```python
from build123d import *

# Parameters (mm, degrees)
BOSS_EXTRUDE1_DEPTH     = 22.5
CUT_EXTRUDE1_DEPTH      = 17.5
SKETCH4_R               = 1
CUT_EXTRUDE2_DEPTH      = 15
CUT_EXTRUDE2_DEPTH_BACK = 12.5
SKETCH5_W               = 10.5
SKETCH5_H               = 12.5
CUT_EXTRUDE3_DEPTH      = 20
SKETCH6_R               = 1.4
CUT_EXTRUDE4_DEPTH      = 10
SKETCH8_R               = 1
SKETCH8_W               = 24
SKETCH8_H               = 13
CUT_EXTRUDE6_DEPTH      = 6
SKETCH9_R               = 1.5
CUT_EXTRUDE7_DEPTH      = 23.5
SKETCH10_R              = 3
CUT_EXTRUDE8_DEPTH      = 5
SKETCH14_W              = 12
SKETCH14_H              = 17.5
BOSS_EXTRUDE3_DEPTH     = 3.5
SKETCH11_R              = 1.5
CUT_EXTRUDE9_DEPTH      = 10
SKETCH16_R              = 2
CUT_EXTRUDE11_DEPTH     = 2
SKETCH18_W              = 6.5
SKETCH18_H              = 2.5
CUT_EXTRUDE12_DEPTH     = 23.5
CUT_EXTRUDE14_DEPTH     = 35
SKETCH22_R              = 1.6
CUT_EXTRUDE15_DEPTH     = 23.5
SKETCH23_R              = 3
CUT_EXTRUDE18_DEPTH     = 3
SKETCH25_W              = 5
SKETCH25_H              = 11.5
BOSS_EXTRUDE4_DEPTH     = 2


with BuildPart() as part:
    # Sketch2 → Boss-Extrude1 (new body)
    with BuildSketch(Plane(origin=(0, 0, 0), x_dir=(1, 0, 0), z_dir=(0, 1, 0))):
        with BuildLine():
            Line((0, 0), (46, 0))
            ThreePointArc((46, 0), (53.071067812, 2.928932188), (56, 10))
            Line((56, 10), (56, 24))
            ThreePointArc((56, 24), (53.071067812, 31.071067812), (46, 34))
            Line((46, 34), (0, 34))
            Line((0, 34), (0, 14))
            Line((0, 14), (-6.5, 14))
            Line((-6.5, 14), (-6.5, 0))
            Line((-6.5, 0), (0, 0))
        make_face()
    extrude(amount=BOSS_EXTRUDE1_DEPTH)

    # Sketch3 → Cut-Extrude1 (cut)
    with BuildSketch(Plane(origin=(0, 22.5, 0), x_dir=(1, 0, 0), z_dir=(0, 1, 0))):
        with BuildLine():
            Line((45, 32), (5, 32))
            Line((5, 32), (5, 3.5))
            Line((5, 3.5), (17, 3.5))
            Line((17, 3.5), (17, 2))
            Line((17, 2), (45, 2))
            Line((45, 2), (45, 4))
            ThreePointArc((45, 4), (46.464466094, 7.535533906), (50, 9))
            Line((50, 9), (54, 9))
            Line((54, 9), (54, 25))
            Line((54, 25), (50, 25))
            ThreePointArc((50, 25), (46.464466094, 26.464466094), (45, 30))
            Line((45, 30), (45, 32))
        make_face()
    extrude(amount=-CUT_EXTRUDE1_DEPTH, mode=Mode.SUBTRACT)

    # Sketch4 → Cut-Extrude2 (cut, two sides)
    with BuildSketch(Plane(origin=(5, 0, 0), x_dir=(0, 0, -1), z_dir=(1, 0, 0))) as cut_extrude2_sk:
        with Locations((28.5, 15.25)):
            Circle(SKETCH4_R)
        with Locations((28.5, 7.25)):
            Circle(SKETCH4_R)
        with Locations((16.5, 7.25)):
            Circle(SKETCH4_R)
        with Locations((16.5, 15.25)):
            Circle(SKETCH4_R)
    extrude(amount=CUT_EXTRUDE2_DEPTH, mode=Mode.SUBTRACT)
    extrude(cut_extrude2_sk.sketch, amount=-CUT_EXTRUDE2_DEPTH_BACK, mode=Mode.SUBTRACT)

    # Sketch5 → Cut-Extrude3 (cut)
    with BuildSketch(Plane.ZY.offset(6.5)):
        with Locations((-8.75, 11.5)):
            Rectangle(SKETCH5_W, SKETCH5_H)
    extrude(amount=-CUT_EXTRUDE3_DEPTH, mode=Mode.SUBTRACT)

    # Sketch6 → Cut-Extrude4 (cut)
    with BuildSketch(Plane(origin=(0, 22.5, 0), x_dir=(1, 0, 0), z_dir=(0, 1, 0))):
        with Locations((0.5, 10)):
            Circle(SKETCH6_R)
    extrude(amount=-CUT_EXTRUDE4_DEPTH, mode=Mode.SUBTRACT)

    # Sketch8 → Cut-Extrude6 (cut, through all)
    with BuildSketch(Plane(origin=(0, 5, 0), x_dir=(1, 0, 0), z_dir=(0, 1, 0))):
        with Locations((50.6, 17)):
            Circle(SKETCH8_R)
        with Locations((22.4, 17)):
            Circle(SKETCH8_R)
        with Locations((36.5, 17)):
            Rectangle(SKETCH8_W, SKETCH8_H)
    extrude(amount=-CUT_EXTRUDE6_DEPTH, mode=Mode.SUBTRACT)

    # Sketch9 → Cut-Extrude7 (cut, through all)
    with BuildSketch(Plane(origin=(0, 22.5, 0), x_dir=(1, 0, 0), z_dir=(0, 1, 0))):
        with Locations((49.5, 29)):
            Circle(SKETCH9_R)
        with Locations((49.5, 5)):
            Circle(SKETCH9_R)
    extrude(amount=-CUT_EXTRUDE7_DEPTH, mode=Mode.SUBTRACT)

    # Sketch10 → Cut-Extrude8 (cut)
    with BuildSketch(Plane.XZ):
        with Locations((49.5, -5)):
            Circle(SKETCH10_R)
        with Locations((49.5, -29)):
            Circle(SKETCH10_R)
    extrude(amount=-CUT_EXTRUDE8_DEPTH, mode=Mode.SUBTRACT)

    # Sketch14 → Boss-Extrude3 (add, symmetric)
    with BuildSketch(Plane.XY.offset(-22.5)):
        with Locations((11, 13.75)):
            Rectangle(SKETCH14_W, SKETCH14_H)
    extrude(amount=BOSS_EXTRUDE3_DEPTH, both=True)

    # Sketch11 → Cut-Extrude9 (cut)
    with BuildSketch(Plane.XZ):
        with Locations((8, -8)):
            Circle(SKETCH11_R)
        with Locations((8, -26)):
            Circle(SKETCH11_R)
    extrude(amount=-CUT_EXTRUDE9_DEPTH, mode=Mode.SUBTRACT)

    # Sketch16 → Cut-Extrude11 (cut)
    with BuildSketch(Plane(origin=(5, 0, 0), x_dir=(0, 0, -1), z_dir=(1, 0, 0))):
        with Locations((28.5, 15.25)):
            Circle(SKETCH16_R)
        with Locations((28.5, 7.25)):
            Circle(SKETCH16_R)
        with Locations((16.5, 7.25)):
            Circle(SKETCH16_R)
        with Locations((16.5, 15.25)):
            Circle(SKETCH16_R)
    extrude(amount=-CUT_EXTRUDE11_DEPTH, mode=Mode.SUBTRACT)

    # Sketch18 → Cut-Extrude12 (cut, through all)
    with BuildSketch(Plane(origin=(0, 22.5, 0), x_dir=(1, 0, 0), z_dir=(0, 1, 0))):
        with Locations((-3.25, 1.25)):
            Rectangle(SKETCH18_W, SKETCH18_H)
    extrude(amount=-CUT_EXTRUDE12_DEPTH, mode=Mode.SUBTRACT)

    # Sketch21 → Cut-Extrude14 (cut, through all)
    with BuildSketch(Plane.XY):
        Polygon((5, 22.5), (56, 11.25), (56, 22.5), align=None)
    extrude(amount=-CUT_EXTRUDE14_DEPTH, mode=Mode.SUBTRACT)

    # Sketch22 → Cut-Extrude15 (cut, through all)
    with BuildSketch(Plane.XZ):
        with Locations((14, -22.5)):
            Circle(SKETCH22_R)
    extrude(amount=-CUT_EXTRUDE15_DEPTH, mode=Mode.SUBTRACT)

    # Sketch23 → Cut-Extrude18 (cut)
    with BuildSketch(Plane.XZ):
        with Locations((14, -22.5)):
            Circle(SKETCH23_R)
    extrude(amount=-CUT_EXTRUDE18_DEPTH, mode=Mode.SUBTRACT)

    # Sketch25 → Boss-Extrude4 (add)
    with BuildSketch(Plane(origin=(0, 22.5, 0), x_dir=(1, 0, 0), z_dir=(0, 1, 0))):
        with Locations((-4, 8.25)):
            Rectangle(SKETCH25_W, SKETCH25_H)
    extrude(amount=BOSS_EXTRUDE4_DEPTH)


solid = part.part
```
Geometry: final body of the model. Coordinates: model frame, mm. A direction names the side the tool comes from. Round coordinates to 2 decimals unless told otherwise and drop trailing zeros. Loops run counter-clockwise (first coordinate to the right, second up) from the corner with the lowest first, then second, coordinate; pieces in that order, holes last. Notation, with made-up numbers: (20.25, 46.5) -> (35.25, 46.5) arc R33 ccw to (35.25, 84.5) -> close; hole circle Ø7 at (64.5, 50.25). An arc over 180 degrees is marked (long way). Use one line per item in the form item = value. Start each with the question number.
1) Section A-A on x = 38. Output: boundary loops of the cut face in (y, z), then the cut area to 3 significant figures.
2) Draft query along Y for faces 6 (the cylindrical face through (46.5, 2.5, -4.9)), 7 (the cylindrical face through (1.52, 14.36, -16.96)), 8 (the flat face through (-1, 17.75, -9)), 9 (the flat face through (45.49, 13.57, -5.59)). Return one class per face: released by +Y, released by -Y, zero draft, split by the parting line, or undercut.
3) First-contact query: P1, Ø5, axis at x = 15, z = -23, coming from the -Y side; P2, Ø0.6, axis at y = 24, z = -10.5, coming from the +X side; P3, Ø2, axis at x = 11, z = -26.5, coming from the +Y side; P4, Ø1.6, axis at x = 50.6, z = -17, coming from the -Y side. Flat tips, straight axial feed; report the tip coordinate or a pass-through.
4) Section B-B on y = 7.25. Give the number of separate pieces and of enclosed holes in the cut face, then the cut area to 3 significant figures.
5) Line query: L1, parallel to Z at x = 12, y = 5.5; L2, parallel to Z at x = 8, y = 2; L3, parallel to Z at x = 22.4, y = 3.95. Output: solid intervals per line, ascending.
6) Section C-C on z = -22.5. Output: boundary loops of the cut face in (x, y), then the cut area to 3 significant figures.
7) Access query for faces 1 (the flat face through (8, 10, -25)), 2 (the flat face through (48.5, 3, -17)), 3 (the flat face through (2, 11, -14)), 4 (the cylindrical face through (4.014, 8.602, -15.026)), 5 (the flat face through (17, 12, -22)). Directions: +Z, -Z, +X, -X, +Y, -Y. A direction counts if a zero-diameter tool reaches every point of the face in a straight line with its end or side. Return the directions, or none.
8) Section D-D on x = 8. Output: boundary loops of the cut face in (y, z).
Response:
q1.outline = (0, -34) -> (15.22, -34) -> (15.22, -32) -> (5, -32) -> (5, -23.5) -> (0, -23.5) -> close; (0, -10.5) -> (5, -10.5) -> (5, -2) -> (15.22, -2) -> (15.22, 0) -> (0, 0) -> close
q1.area = 146 mm^2
q2.face_6 = zero draft
q2.face_7 = undercut
q2.face_8 = undercut
q2.face_9 = released by +Y
q3.P1 = 0
q3.P2 = -1.5
q3.P3 = 21.37
q3.P4 = through
q4.separate_pieces = 3
q4.enclosed_holes = 3
q4.area = 509 mm^2
q5.L1 = -34 to -32, -26 to -19, -3.5 to 0
q5.L2 = -34 to -27.5, -24.5 to -9.5, -6.5 to 0
q5.L3 = -34 to -18, -16 to 0
q6.outline = (0, 0) -> (11, 0) -> (11, 3) -> (12.4, 3) -> (12.4, 20.87) -> (5, 22.5) -> (0, 22.5) -> close; (15.6, 3) -> (17, 3) -> (17, 0) -> (24.5, 0) -> (24.5, 5) -> (17, 5) -> (17, 19.85) -> (15.6, 20.16) -> close; (48.5, 0) -> (56, 0) -> (56, 11.25) -> (54, 11.69) -> (54, 5) -> (48.5, 5) -> close
q6.area = 381 mm^2
q7.face_1 = -Y
q7.face_2 = +Y, -Y
q7.face_3 = -X
q7.face_4 = none
q7.face_5 = +Y
q8.outline = (0, -34) -> (21.84, -34) -> (21.84, -32) -> (5, -32) -> (5, -27.5) -> (0, -27.5) -> close; (0, -24.5) -> (10, -24.5) -> (10, -26) -> (21.84, -26) -> (21.84, -19) -> (5, -19) -> (5, -9.5) -> (0, -9.5) -> close; (0, -6.5) -> (5, -6.5) -> (5, -3.5) -> (21.84, -3.5) -> (21.84, 0) -> (0, 0) -> close
